Verification items for the finished model (mm, model axes). Give positions to 0.01 mm unless a question says otherwise; leave off trailing zeros. Order: outer loops, then holes, each group sorted by start corner. A loop starts at its lowest first (then second) coordinate and runs counter-clockwise, first axis right, second up. Notation, with made-up numbers: (65.25, -6.5) -> (71.25, -6.5) arc R34 cw to (71.25, 31.5) -> close; hole circle Ø8 at (-33, 86). An arc over 180 degrees is marked (long way). One line per question, with ' | ' between items. Start each with the question number.
Q1. Material ranges on probe 1 along Y at (x, z) = (12, 3.3); probe 2 along Y at (x, z) = (13, 3.3); probe 3 along X at (y, z) = (22, 4.65), recorded low to high. Write a range as [from, to].
Q2. Section check C-C on x = 54. Record the cut outline in (y, z).
Q3. Mould release check, pull along X, two halves, no side actions. Record for faces 1 (the cylindrical face through (49.42, 21.26, 2.96)), 2 (the flat face through (23, 22, 6)), 3 (the flat face through (0, 15, 3)): released by +X, released by -X, zero draft, split by the parting line, or undercut.
Q4. Go/stop test with a flat-tipped pin: pin 1 (1.9 mm diameter, centred on x = 54, y = 15, fed in from -Z). Record where the tip stops, or that it passes through.
Q5. Section check D-D on z = 3. Record the cut outline in (x, y), plus the area to 3 significant figures.
Q6. Section check B-B on y = 15. Record the cut outline in (x, z), plus the area to 3 significant figures.
Q7. Section check A-A on x = 48. Record the cut outline in (y, z).
Autodesk Inventor part; units mm, degrees
ref_plane "YZ Plane" through (0, 0, 0) normal (1, 0, 0) x (0, 1, 0)
ref_plane "XZ Plane" through (0, 0, 0) normal (0, 1, 0) x (-1, 0, 0)
ref_plane "XY Plane" through (0, 0, 0) normal (0, 0, 1) x (1, 0, 0)
sketch "スケッチ1" plane through (0, 0, 0) normal (0, 0, 1) x (1, 0, 0)
  line L0 (0, 0) -> (60, 0)
  line L1 (60, 0) -> (60, 30)
  line L2 (60, 30) -> (0, 30)
  line L3 (0, 30) -> (0, 0)
  dimension "d0" = 60
  dimension "d1" = 30
extrude "押し出し1" add sketch "スケッチ1" along normal blind 6
sketch "スケッチ2" plane through (0, 0, 6) normal (0, 0, 1) x (1, 0, 0)
  circle A0 centre (30, 15) radius 9.5
  line L0 (0, 30) -> (0, 0)
  line L1 (60, 30) -> (0, 30)
  dimension "d4" = 19
  dimension "d5" = 30
  dimension "d6" = 15
extrude "押し出し2" cut sketch "スケッチ2" against normal blind 6
sketch "スケッチ3" plane through (0, 0, 6) normal (0, 0, 1) x (1, 0, 0)
  circle A0 centre (12, 22) radius 1.6
  circle A1 centre (12, 8) radius 1.6
  line L0 (60, 30) -> (0, 30)
  line L1 (0, 0) -> (60, 0)
  line L2 (0, 30) -> (0, 0)
  circle A2 centre (6, 15) radius 1.6
  line L3 (30, 30) -> (30, 0) construction
  line L4 (0, 0) -> (60, 0)
  circle A3 centre (48, 22) radius 1.6
  circle A4 centre (48, 8) radius 1.6
  circle A5 centre (54, 15) radius 1.6
  dimension "d9" = 3.2
  dimension "d10" = 3.2
  dimension "d11" = 8
  dimension "d12" = 8
  dimension "d13" = 12
  dimension "d14" = 12
  dimension "d15" = 3.2
  dimension "d16" = 15
  dimension "d17" = 6
hole "穴1" at (12, 22, 6) at (6, 15, 6) at (12, 8, 6) at (48, 22, 6) at (54, 15, 6) at (48, 8, 6) direction (0, 0, -1) diameter 3.2 depth 6
equation "\"BendRadius\" = Thickness"
equation "\"BendReliefWidth\" = Thickness"
equation "\"BendReliefDepth\" = 0.5 * Thickness"
equation "\"CornerReliefSize\" = 4 * Thickness"
equation "\"MinimumRemnant\" = 2 * Thickness"
equation "\"TransitionRadius\" = BendRadius"
equation "\"JacobiRadiusSize\" = BendRadius"
equation "\"GapSize\" = Thickness"
properties part number "nhk45"
Filled in:
1) probe 1: [0, 6.4], [9.6, 20.4], [23.6, 30] | probe 2: [0, 6.75], [9.25, 20.75], [23.25, 30] | probe 3: [0, 10.4], [13.6, 23.58], [36.42, 46.4], [49.6, 60]
2) outline: (0, 0) -> (13.4, 0) -> (13.4, 6) -> (0, 6) -> close; (16.6, 0) -> (30, 0) -> (30, 6) -> (16.6, 6) -> close
3) face 1: undercut | face 2: zero draft | face 3: released by -X
4) pin 1: through
5) outline: (0, 0) -> (60, 0) -> (60, 30) -> (0, 30) -> close; hole circle Ø3.2 at (6, 15); hole circle Ø3.2 at (12, 8); hole circle Ø3.2 at (12, 22); hole circle Ø19 at (30, 15); hole circle Ø3.2 at (48, 8); hole circle Ø3.2 at (48, 22); hole circle Ø3.2 at (54, 15) | area: 1,470 mm²
6) outline: (0, 0) -> (4.4, 0) -> (4.4, 6) -> (0, 6) -> close; (7.6, 0) -> (20.5, 0) -> (20.5, 6) -> (7.6, 6) -> close; (39.5, 0) -> (52.4, 0) -> (52.4, 6) -> (39.5, 6) -> close; (55.6, 0) -> (60, 0) -> (60, 6) -> (55.6, 6) -> close | area: 208 mm²
7) outline: (0, 0) -> (6.4, 0) -> (6.4, 6) -> (0, 6) -> close; (9.6, 0) -> (20.4, 0) -> (20.4, 6) -> (9.6, 6) -> close; (23.6, 0) -> (30, 0) -> (30, 6) -> (23.6, 6) -> close
